The model under review builds one solid part; all positions refer to its coordinate system, in mm. Coordinates: 2 decimals unless noted, no trailing zeros. Loops run counter-clockwise (first coordinate to the right, second up) from the corner with the lowest first, then second, coordinate; pieces in that order, holes last. Notation, with made-up numbers: M 8,59 L 58,59 A24 cw 58,87 Z; hole C 73.5,6 d9. An arc over 180 degrees is marked long. One line per item, written item: value.
Autodesk Inventor part; units mm, degrees
ref_plane "YZ Plane" through (0, 0, 0) normal (1, 0, 0) x (0, 1, 0)
ref_plane "XZ Plane" through (0, 0, 0) normal (0, 1, 0) x (-1, 0, 0)
ref_plane "XY Plane" through (0, 0, 0) normal (0, 0, 1) x (1, 0, 0)
sketch "Esboço1" plane through (0, 0, 0) normal (0, 1, 0) x (-1, 0, 0)
  line L0 (0, 0) -> (3.5, 0)
  line L1 (4, -2) -> (5, -2)
  line L2 (5.5, 0) -> (7.5, 0)
  line L3 (7.5, 0) -> (7.5, -12)
  line L4 (7.5, -12) -> (5.5, -12)
  line L5 (5, -10) -> (4, -10)
  line L6 (3.5, -12) -> (0, -12)
  line L7 (0, -12) -> (0, 0)
  line L8 (5.5, 0) -> (5, -2)
  line L9 (3.5, 0) -> (4, -2)
  line L10 (5, -10) -> (5.5, -12)
  line L11 (3.5, -12) -> (4, -10)
  dimension "d0" = 7.5
  dimension "d1" = 12
  dimension "d2" = 8
  dimension "d3" = 1
  dimension "d4" = 3.5
  dimension "d5" = 0.5
extrude "Extrusão1" add sketch "Esboço1" along normal blind 469
sketch "Esboço2" plane through (-7.5, 0, -12) normal (-1, 0, 0) x (0, 0, 1)
  line L0 (0, 0) -> (0, 469)
  line L1 (0, 0) -> (12, 0)
  line L2 (12, 0) -> (12, 469)
  line L3 (12, 0) -> (0, 0)
  point P0 (6, 7.7)
  point P1 (6, 32.9)
  point P2 (6, 58.1)
  point P3 (6, 83.3)
  point P4 (6, 108.5)
  point P5 (6, 133.7)
  point P6 (6, 158.9)
  point P7 (6, 184.1)
  point P8 (6, 209.3)
  point P9 (6, 234.5)
  point P10 (6, 259.7)
  point P11 (6, 284.9)
  point P12 (6, 310.1)
  point P13 (6, 335.3)
  point P14 (6, 360.5)
  point P15 (6, 385.7)
  point P16 (6, 410.9)
  point P17 (6, 436.1)
  point P18 (6, 0)
  point P19 (6, 461.3)
  point P20 (6, 0)
  dimension "d10" = 25.2
  dimension "d18" = 6
  dimension "d27" = 453.6
  dimension "d28" = 469
  dimension "d29" = 7.7
hole "Furo1" at (-7.5, 7.7, -6) at (-7.5, 32.9, -6) at (-7.5, 58.1, -6) at (-7.5, 83.3, -6) at (-7.5, 108.5, -6) at (-7.5, 133.7, -6) at (-7.5, 158.9, -6) at (-7.5, 184.1, -6) at (-7.5, 209.3, -6) at (-7.5, 234.5, -6) at (-7.5, 259.7, -6) at (-7.5, 284.9, -6) at (-7.5, 310.1, -6) at (-7.5, 335.3, -6) at (-7.5, 360.5, -6) at (-7.5, 385.7, -6) at (-7.5, 410.9, -6) at (-7.5, 436.1, -6) at (-7.5, 461.3, -6) direction (1, 0, 0) diameter 3 depth 7.5 counterbore diameter 4 counterbore depth 2
equation "\"d24\" = Espessura"
equation "\"Raio_vergadura\" = Espessura"
equation "\"Largura_alívio_de_vergadura\" = Espessura"
equation "\"Profundidade_alívio_de_vergadura\" = 0.5 * Espessura"
equation "\"Tamanho_alívio_de_dobra\" = 4 * Espessura"
equation "\"Remanescente_mínimo\" = 2 * Espessura"
equation "\"Raiodetransição\" = Raio_vergadura"
equation "\"Tamanho_de_raio_de_Jacobi\" = Raio_vergadura"
equation "\"TamanhoFolga\" = Espessura"
properties part number "Trilho" material "Aço inoxidável"
(1) Insertion check: pin 1 Ø5 at (y, z) = (7.7, -6) entering from +X; pin 2 Ø2 at (y, z) = (158.5, -5.5) entering from -X; pin 3 Ø0.5 at (x, y) = (-4.5, 282) entering from +Z. Each pin has a flat end and moves straight along its axis. Give the tip position at first contact, or say it passes through.
Checks:
pin 1: x = 0
pin 2: x = -5.5
pin 3: z = -2
(2) Add section A-A on x = -2. State how many separate pieces and enclosed holes the cut face has, then the cut area to 3 significant figures.
Checks:
separate pieces: 1
enclosed holes: 19
area: 5,490 mm^2
(3) Add section B-B on y = 351.5. State the section outline as (x, z) points.
Checks:
outline: M -7.5,-12 L -5.5,-12 L -5,-10 L -4,-10 L -3.5,-12 L 0,-12 L 0,0 L -3.5,0 L -4,-2 L -5,-2 L -5.5,0 L -7.5,0 Z
(4) To check wall thickness, follow L1, parallel to Z at x = -2.3, y = 284.9; L2, parallel to Z at x = -4.35, y = 259.7; L3, parallel to X at y = 384, z = -10.5 (3 decimals). State the ranges of each line that lie inside material, in increasing order. Write a range as [from, to].
Checks:
L1: [-12, -7.5], [-4.5, 0]
L2: [-10, -7.5], [-4.5, -2]
L3: [-7.5, -5.125], [-3.875, 0]
